```python
from build123d import *

# Parameters (mm, degrees)
F1_DEPTH = 0.78
F2_R     = 0.5
F4_DEPTH = 0.7


with BuildPart() as f1:
    # F0 (on Front) → F1 (new body)
    with BuildSketch(Plane.XZ):
        Polygon((4.2184664682, 12.45), (-7.45, 12.45), (-7.45, -12.45), (7.45, -12.45), (7.45, 9.2184664682), align=None)
    extrude(amount=F1_DEPTH)

    # F2
    f2_edges = [f1.edges().sort_by_distance(p)[0] for p in [
        (-7.45, -0.39, 12.45),
        (-7.45, -0.39, -12.45),
        (7.45, -0.39, -12.45),
        (7.45, -0.39, 9.218466),
        (4.218466, -0.39, 12.45),
    ]]
    fillet(f2_edges, radius=F2_R)

    # F3 (on face) → F4 (cut)
    with BuildSketch(Plane.XZ.offset(0.78)):
        Polygon((3.7478837054, 5.17), (-6.65, 5.17), (-6.65, -9.83), (5.45, -9.83), (5.45, 3.4678837054), align=None)
    extrude(amount=-F4_DEPTH, mode=Mode.SUBTRACT)


solid = f1.part
```
Part model, mm, in its own coordinate system. Round coordinates to 2 decimals unless told otherwise and drop trailing zeros. Loops run counter-clockwise (first coordinate to the right, second up) from the corner with the lowest first, then second, coordinate; pieces in that order, holes last. Notation, with made-up numbers: (-3.5, 54) -> (49.5, 54) arc R32 ccw to (49.5, 87) -> close; hole circle Ø4 at (-15.5, 65.5). An arc over 180 degrees is marked (long way). Use a Markdown table: item, result.
1) Cut at A-A, the plane y = -0.3. List the corners of the cut face in (x, z), and give its area (3 significant figures).
The answers:
| item | result |
|---|---|
| outline | (-7.45, -11.95) arc R0.5 ccw to (-6.95, -12.45) -> (6.95, -12.45) arc R0.5 ccw to (7.45, -11.95) -> (7.45, 9.01) arc R0.5 ccw to (7.3, 9.36) -> (4.36, 12.3) arc R0.5 ccw to (4.01, 12.45) -> (-6.95, 12.45) arc R0.5 ccw to (-7.45, 11.95) -> close; hole (-6.65, -9.83) -> (5.45, -9.83) -> (5.45, 3.47) -> (3.75, 5.17) -> (-6.65, 5.17) -> close |
| area | 186 mm2 |
2) Cut at B-B, the plane x = -5.5. List the corners of the cut face in (y, z), and give its area (3 significant figures).
The answers:
| item | result |
|---|---|
| outline | (-0.78, -12.45) -> (0, -12.45) -> (0, 12.45) -> (-0.78, 12.45) -> (-0.78, 5.17) -> (-0.08, 5.17) -> (-0.08, -9.83) -> (-0.78, -9.83) -> close |
| area | 8.92 mm2 |
3) Cut at C-C, the plane z = -2.5. List the corners of the cut face in (x, y).
The answers:
| item | result |
|---|---|
| outline | (-7.45, -0.78) -> (-6.65, -0.78) -> (-6.65, -0.08) -> (5.45, -0.08) -> (5.45, -0.78) -> (7.45, -0.78) -> (7.45, 0) -> (-7.45, 0) -> close |
4) Cut at D-D, the plane x = 6.25. List the corners of the cut face in (y, z).
The answers:
| item | result |
|---|---|
| outline | (-0.78, -12.45) -> (0, -12.45) -> (0, 10.42) -> (-0.78, 10.42) -> close |
5) Pull direction X, two halves, no side cores. Call faces 1 (the flat face through (4.61, -0.43, 4.31)), 2 (the flat face through (0, -0.78, 6)), 3 (the flat face through (5.855, -0.385, 10.814)): pulls with the +X half, pulls with the -X half, needs draft (parallel to the pull), parting line crosses it, or undercut.
The answers:
| item | result |
|---|---|
| face 1 | undercut |
| face 2 | needs draft |
| face 3 | pulls with the +X half |
6) Probe line 1 (X direction, y = -0.65, z = -7.5); line 2 (Z direction, x = -2.75, y = -0.3); line 3 (X direction, y = -0.5, z = 4.25). List the from-to ranges inside material, lowest first. Write a range as [from, to].
The answers:
| item | result |
|---|---|
| line 1 | x = [-7.45, -6.65], [5.45, 7.45] |
| line 2 | z = [-12.45, -9.83], [5.17, 12.45] |
| line 3 | x = [-7.45, -6.65], [4.67, 7.45] |
7) Drop a flat-ended pin along its axis: pin 1 Ø6 at (x, z) = (-3.5, -3) entering from -Y. Give the stop position or say it passes through.
The answers:
| item | result |
|---|---|
| pin 1 | stops at y = -0.08 |
